```python
from build123d import *

# Parameters (mm, degrees)
CROQUIS1_W              = 43.5
CROQUIS1_H              = 43.5
CROQUIS1_R              = 1.5
SALIENTE_EXTRUIR1_DEPTH = 1
CROQUIS2_W              = 23
CROQUIS2_H              = 16
SALIENTE_EXTRUIR2_DEPTH = 21
CROQUIS3_W              = 24.693378616
CROQUIS3_H              = 16.159035638
SALIENTE_EXTRUIR3_DEPTH = 11
CHAFL_N1_SIZE           = 7
CHAFL_N1_SIZE2          = 10


with BuildPart() as part:
    # Croquis1 → Saliente-Extruir1 (new body)
    with BuildSketch(Plane(origin=(0, 0, 0), x_dir=(1, 0, 0), z_dir=(0, 1, 0))):
        Rectangle(CROQUIS1_W, CROQUIS1_H)
        with Locations((-18.75, 18.75)):
            Circle(CROQUIS1_R, mode=Mode.SUBTRACT)
        with Locations((18.75, 18.75)):
            Circle(CROQUIS1_R, mode=Mode.SUBTRACT)
        with Locations((18.75, -18.75)):
            Circle(CROQUIS1_R, mode=Mode.SUBTRACT)
        with Locations((-18.75, -18.75)):
            Circle(CROQUIS1_R, mode=Mode.SUBTRACT)
    extrude(amount=SALIENTE_EXTRUIR1_DEPTH)

    # Croquis2 → Saliente-Extruir2 (add)
    with BuildSketch(Plane(origin=(0, 1, 0), x_dir=(1, 0, 0), z_dir=(0, 1, 0))):
        with Locations((0, 13.75)):
            Rectangle(CROQUIS2_W, CROQUIS2_H)
    extrude(amount=SALIENTE_EXTRUIR2_DEPTH)

    # Croquis3 → Saliente-Extruir3 (add)
    with BuildSketch(Plane(origin=(0, 1, 0), x_dir=(1, 0, 0), z_dir=(0, 1, 0))):
        with Locations((0, -9.671859961)):
            Rectangle(CROQUIS3_W, CROQUIS3_H)
    extrude(amount=SALIENTE_EXTRUIR3_DEPTH)

    # Chaflán1
    chafl_n1_edges = [part.edges().sort_by_distance(p)[0] for p in [
        (0, 22, -5.75),
    ]]
    chafl_n1_side = [part.faces().sort_by_distance(p)[0] for p in [
        (0, 11.5, -5.75),
    ]]
    chamfer(chafl_n1_edges, length=CHAFL_N1_SIZE, length2=CHAFL_N1_SIZE2, reference=chafl_n1_side[0])


solid = part.part
```
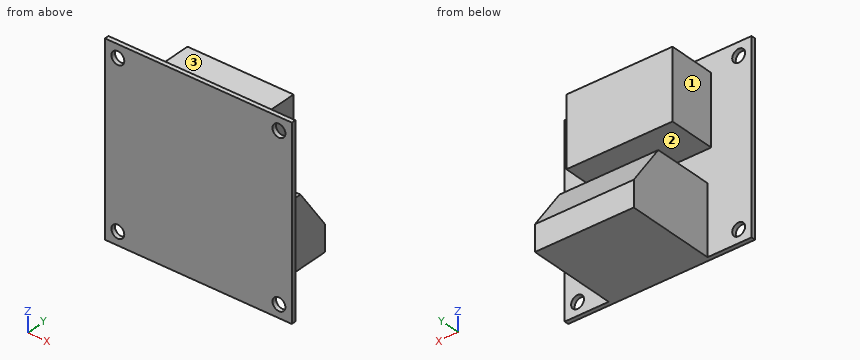
Check sheet for the modelled part. Datum: model origin and axes. Units: mm. Face numbers are marked on the shaded views. A direction names the side the tool comes from. Coordinates: 2 decimals unless noted, no trailing zeros. Order: outer loops, then holes, each group sorted by start corner. A loop starts at its lowest first (then second) coordinate and runs counter-clockwise, first axis right, second up. Notation, with made-up numbers: M -21.5,-36 L 0.5,-36 A8 ccw 0.5,-31 Z; hole C 87.25,65.25 d6. An arc over 180 degrees is marked long. Write each question's results on one line, items separated by ' | '. Start each with the question number.
1. Go/stop test with flat-tipped pins: P1, Ø9, axis at y = 6, z = 7, coming from the -X side; P2, Ø8, axis at y = 17, z = -8, coming from the +X side; P3, Ø6, axis at y = 16, z = -10.5, coming from the -X side. Record where each tip stops, or that it passes through.
2. Access from +Z, -Z, +X, -X, +Y, -Y to the whole of each face (thin tool, end or side, straight path). Record for the marked faces 1, 2 and 3.
3. Material ranges on probe 1 along Z at (x, y) = (18.75, 0.4); probe 2 along Z at (x, y) = (1, 8), recorded low to high.
4. Cross-section at B-B on y = 5.5. Record the cut outline in (x, z).
5. Cross-section at A-A on z = -18.75. Record the cut outline in (x, y).
6. Cross-section at D-D on z = 18.75. Record the cut outline in (x, y).
7. Cross-section at C-C on x = 18.75. Record the cut outline in (y, z), and give its area (3 significant figures).
Checks:
1) P1: stops at x = -12.35 | P2: stops at x = 11.5 | P3: stops at x = -11.5
2) face 1: +Z, -Z, -X, +Y | face 2: +X, -X, +Y | face 3: +Z, +X, -X, +Y
3) probe 1: z = -21.75 to -20.25, -17.25 to 17.25, 20.25 to 21.75 | probe 2: z = -21.75 to -5.75, 1.59 to 17.75
4) outline: M -12.35,1.59 L 12.35,1.59 L 12.35,17.75 L -12.35,17.75 Z; M -11.5,-21.75 L 11.5,-21.75 L 11.5,-5.75 L -11.5,-5.75 Z
5) outline: M -21.75,0 L -20.25,0 L -20.25,1 L -21.75,1 Z; M -17.25,0 L 17.25,0 L 17.25,1 L 11.5,1 L 11.5,22 L -11.5,22 L -11.5,1 L -17.25,1 Z; M 20.25,0 L 21.75,0 L 21.75,1 L 20.25,1 Z
6) outline: M -21.75,0 L -20.25,0 L -20.25,1 L -21.75,1 Z; M -17.25,0 L 17.25,0 L 17.25,1 L -17.25,1 Z; M 20.25,0 L 21.75,0 L 21.75,1 L 20.25,1 Z
7) outline: M 0,-21.75 L 1,-21.75 L 1,-20.25 L 0,-20.25 Z; M 0,-17.25 L 1,-17.25 L 1,17.25 L 0,17.25 Z; M 0,20.25 L 1,20.25 L 1,21.75 L 0,21.75 Z | area: 37.5 mm²
